The model under review builds one solid part; all positions refer to its coordinate system, in mm. A direction names the side the tool comes from. Coordinates: 2 decimals unless noted, no trailing zeros. Loops run counter-clockwise (first coordinate to the right, second up) from the corner with the lowest first, then second, coordinate; pieces in that order, holes last. Notation, with made-up numbers: M 63.5,-1.75 L 78.5,-1.75 A9 cw 78.5,3.25 Z; hole C -15.5,53 d8. An arc over 180 degrees is marked long. One line per item, written item: value.
Autodesk Inventor part; units mm, degrees
ref_plane "YZ Plane" through (0, 0, 0) normal (1, 0, 0) x (0, 1, 0)
ref_plane "XZ Plane" through (0, 0, 0) normal (0, 1, 0) x (-1, 0, 0)
ref_plane "XY Plane" through (0, 0, 0) normal (0, 0, 1) x (1, 0, 0)
sketch "Esboço1" plane through (0, 0, 0) normal (0, 1, 0) x (-1, 0, 0)
  line L0 (0, 0) -> (-91, 0)
  line L1 (-91, 0) -> (-91, -111)
  line L2 (-91, -111) -> (0, -111)
  line L3 (0, -111) -> (0, 0)
  line L4 (-3, -108) -> (-88, -108)
  line L5 (-88, -108) -> (-88, -3)
  line L6 (-88, -3) -> (-3, -3)
  line L7 (-3, -3) -> (-3, -108)
  dimension "d0" = 3
  dimension "d1" = 3
  dimension "d2" = 3
  dimension "d3" = 3
  dimension "d4" = 85
  dimension "d5" = 105
extrude "Extrusão1" add sketch "Esboço1" along normal blind 3 contours L4 L5 L6 L7
extrude "Extrusão2" add sketch "Esboço1" along normal blind 25
sketch "Esboço2" plane through (0, 0, 0) normal (0, 0, 1) x (1, 0, 0)
  circle A0 centre (20, 12) radius 3
  circle A1 centre (66, 13) radius 3.75
  line L0 (0, 0) -> (0, 25)
  line L1 (91, 0) -> (91, 25)
  line L2 (0, 0) -> (91, 0)
  point P0 (0, 12.5)
  dimension "d10" = 6
  dimension "d11" = 7.5
  dimension "d25" = 20
  dimension "d26" = 25
  dimension "d30" = 13
  dimension "d31" = 12
extrude "Extrusão3" cut sketch "Esboço2" against normal blind 30
sketch "Esboço3" plane through (91, 0, 0) normal (1, 0, 0) x (0, 0, -1)
  circle A0 centre (16.1671, 10) radius 1.5
  circle A1 centre (34.0898, 10) radius 1.5
  circle A2 centre (25.3707, 10) radius 1.5
  line L0 (0, 0) -> (111, 0)
  dimension "d14" = 3
  dimension "d15" = 3
  dimension "d16" = 3
  dimension "d32" = 10
  dimension "d33" = 10
  dimension "d34" = 10
extrude "Extrusão4" cut sketch "Esboço3" against normal blind 10
sketch "Esboço4" plane through (0, 3, 0) normal (0, 1, 0) x (1, 0, 0)
  line L0 (29.6, 81.6) -> (63, 81.6)
  line L1 (63, 81.6) -> (63, 98)
  line L2 (63, 98) -> (29.6, 98)
  line L3 (29.6, 98) -> (29.6, 81.6)
  line L4 (88, 108) -> (88, 3)
  line L5 (3, 108) -> (88, 108)
  line L6 (29.6, 81.6) -> (45, 81.6)
  line L7 (45, 81.6) -> (45, 79.6)
  line L8 (45, 79.6) -> (29.6, 79.6)
  line L9 (29.6, 79.6) -> (29.6, 81.6)
  point P0 (0, 0)
  point P1 (63, 89.8)
  dimension "d19" = 33.4
  dimension "d20" = 16.4
  dimension "d23" = 25
  dimension "d24" = 10
  dimension "d35" = 18.4
  dimension "d36" = 15.4
extrude "Extrusão5" cut sketch "Esboço4" against normal blind 1.5
properties part number "Caixa_3DPrint"
(1) Add section C-C on x = 49. State the section outline as (y, z) points, then the cut area to 3 significant figures.
Checks:
outline: M 0,-111 L 25,-111 L 25,-108 L 3,-108 L 3,-98 L 1.5,-98 L 1.5,-81.6 L 3,-81.6 L 3,-3 L 25,-3 L 25,0 L 0,0 Z
area: 440 mm^2
(2) Insertion check: pin 1 Ø2.5 at (y, z) = (10, -16.17) entering from +X; pin 2 Ø20 at (x, z) = (52.5, -91.5) entering from +Y. Each pin has a flat end and moves straight along its axis. Give the tip position at first contact, or say it passes through.
Checks:
pin 1: x = 3
pin 2: y = 3
(3) Tool access review of faces 1 (the face through (46, 14, -3)), 2 (the face through (46, 12, -111)), 3 (the face through (17, 12, -1)), 4 (the face through (89.52, 10.45, -17.6)): name each direction out of +Z, -Z, +X, -X, +Y, -Y from which nothing blocks a thin tool from reaching the whole face with its end or side.
Checks:
face 1: +Y
face 2: -Z, +X, -X, +Y, -Y
face 3: +Z
face 4: +X
(4) Add section D-D on z = -43.5. State the section outline as (x, y) points.
Checks:
outline: M 0,0 L 91,0 L 91,25 L 88,25 L 88,3 L 3,3 L 3,25 L 0,25 Z
(5) Add section A-A on x = 20. State the section outline as (y, z) points, then the cut area to 3 significant figures.
Checks:
outline: M 0,-111 L 25,-111 L 25,-108 L 3,-108 L 3,-3 L 9,-3 L 9,0 L 0,0 Z; M 15,-3 L 25,-3 L 25,0 L 15,0 Z
area: 447 mm^2
(6) Draft analysis for pull direction Y (two halves, no side actions). For faces 5 (the face through (90, 25, -55)), 6 (the face through (0, 12, -56)), 7 (the face through (69.577, 14.126, -1.479)), 8 (the face through (89.52, 10.45, -35.52)), state which applies: pulls with the +Y half, pulls with the -Y half, needs draft (parallel to the pull), parting line crosses it, or undercut.
Checks:
face 5: pulls with the +Y half
face 6: needs draft
face 7: undercut
face 8: undercut
(7) Add section B-B on y = 18.75. State the section outline as (x, z) points, then the cut area to 3 significant figures.
Checks:
outline: M 0,-111 L 91,-111 L 91,0 L 0,0 Z; hole M 3,-108 L 88,-108 L 88,-3 L 3,-3 Z
area: 1,180 mm^2
(8) To check wall thickness, follow L1, parallel to Z at x = 25, y = 18.25; L2, parallel to X at y = 15.5, z = -101.5; L3, parallel to Y at x = 66, z = -1. State the ranges of each line that lie inside material, in increasing order. Write a range as [from, to].
Checks:
L1: [-111, -108], [-3, 0]
L2: [0, 3], [88, 91]
L3: [0, 9.25], [16.75, 25]
